Check sheet for the modelled part. Datum: model origin and axes. Units: mm. Face numbers are marked on the shaded views. Coordinates: 2 decimals unless noted, no trailing zeros. Write each loop counter-clockwise with the first axis right and the second up, starting at its lowest first coordinate (ties: lowest second). Pieces come first, ordered by that corner, then holes. Notation, with made-up numbers: (-11.5, -1.5) - (44.5, -1.5) arc R28 ccw to (44.5, 18.5) - close; hole circle Ø10 at (31, -14). An arc over 180 degrees is marked (long way). Write each question's results on one line, items separated by ' | '.
from build123d import *

# Parameters (mm, degrees)
CROQUIS1_R              = 50
CROQUIS1_R_2            = 45
SALIENTE_EXTRUIR1_DEPTH = 400
CROQUIS2_R              = 55
SALIENTE_EXTRUIR2_DEPTH = 30
SALIENTE_EXTRUIR3_START = -30
CROQUIS3_R              = 55
SALIENTE_EXTRUIR3_DEPTH = 30
CROQUIS4_R              = 12.75
CORTAR_EXTRUIR1_DEPTH   = 179
CROQUIS5_R              = 7.5
CROQUIS5_R_2            = 5
CROQUIS5_R_3            = 12.7
CORTAR_EXTRUIR2_DEPTH   = 60


with BuildPart() as part:
    # Croquis1 → Saliente-Extruir1 (new body)
    with BuildSketch(Plane.XY):
        Circle(CROQUIS1_R)
        Circle(CROQUIS1_R_2, mode=Mode.SUBTRACT)
    extrude(amount=SALIENTE_EXTRUIR1_DEPTH)

    # Croquis2 → Saliente-Extruir2 (add)
    with BuildSketch(Plane.XY):
        Circle(CROQUIS2_R)
    extrude(amount=SALIENTE_EXTRUIR2_DEPTH)

    # Croquis3 → Saliente-Extruir3 (add)
    with BuildSketch(Plane.XY.offset(400).offset(SALIENTE_EXTRUIR3_START)):
        Circle(CROQUIS3_R)
    extrude(amount=SALIENTE_EXTRUIR3_DEPTH)

    # Croquis4 → Cortar-Extruir1 (cut)
    with BuildSketch(Plane(origin=(0, 0, 0), x_dir=(0, 0, -1), z_dir=(1, 0, 0))):
        with Locations(Location((-200, 0, 0), (0, 0, 180))):
            Circle(CROQUIS4_R)
    extrude(amount=-CORTAR_EXTRUIR1_DEPTH, mode=Mode.SUBTRACT)

    # Croquis5 → Cortar-Extruir2 (cut)
    with BuildSketch(Plane(origin=(0, 50, 0), x_dir=(1, 0, 0), z_dir=(0, 1, 0))):
        with Locations(Location((0, -240, 0), (0, 0, 270))):
            Circle(CROQUIS5_R)
        with Locations(Location((0, -160, 0), (0, 0, 270))):
            Circle(CROQUIS5_R)
        with Locations(Location((0, -200, 0), (0, 0, 270))):
            Circle(CROQUIS5_R_2)
        with Locations(Location((0, -350, 0), (0, 0, 270))):
            Circle(CROQUIS5_R_3)
        with Locations(Location((0, -50, 0), (0, 0, 270))):
            Circle(CROQUIS5_R_3)
    extrude(amount=-CORTAR_EXTRUIR2_DEPTH, mode=Mode.SUBTRACT)


solid = part.part
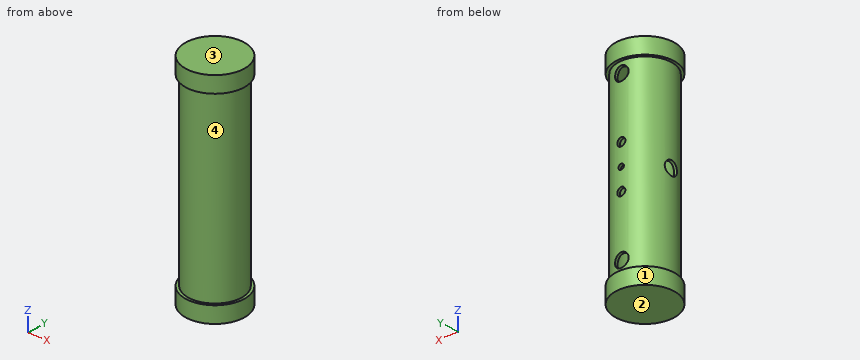
1. Draft check along Z on the marked faces 1, 2, 3 and 4. Enter one of: pulls with the +Z half, pulls with the -Z half, needs draft (parallel to the pull), parting line crosses it, or undercut.
Values follow:
face 1: needs draft | face 2: pulls with the -Z half | face 3: pulls with the +Z half | face 4: undercut
2. Sectioned sample at D-D (z = 98). Record the cut outline in (x, y), then the cut area to 3 significant figures.
Values follow:
outline: circle Ø100 at (0, 0); hole circle Ø90 at (0, 0) | area: 1,490 mm^2
3. Go/stop test with flat-tipped pins: pin 1 (8 mm diameter, centred on x = 0, z = 200, fed in from +Y); pin 2 (12 mm diameter, centred on x = 0, z = 160, fed in from +Y); pin 3 (12 mm diameter, centred on x = -10, y = 29, fed in from -Z); pin 4 (12 mm diameter, centred on y = 42.5, z = 253.5, fed in from +X). Record where each tip stops, or that it passes through.
Values follow:
pin 1: stops at y = -44.82 | pin 2: stops at y = -44.6 | pin 3: stops at z = 0 | pin 4: stops at x = 34.17
4. Sectioned sample at A-A (z = 200). Record the cut outline in (x, y), then the cut area to 3 significant figures.
Values follow:
outline: (-48.35, -12.75) arc R50 ccw (long way) to (5, 49.75) - (5, 44.72) arc R45 cw (long way) to (-43.16, -12.75) - close; (-48.35, 12.75) - (-43.16, 12.75) arc R45 cw to (-5, 44.72) - (-5, 49.75) arc R50 ccw to start | area: 1,310 mm^2
5. Sectioned sample at B-B (y = 21). Record the cut outline in (x, z), then the cut area to 3 significant figures.
Values follow:
outline: (-50.83, 0) - (50.83, 0) - (50.83, 30) - (45.38, 30) - (45.38, 370) - (50.83, 370) - (50.83, 400) - (-50.83, 400) - (-50.83, 370) - (-45.38, 370) - (-45.38, 30) - (-50.83, 30) - close; hole (-39.8, 30) - (39.8, 30) - (39.8, 370) - (-39.8, 370) - close | area: 9,890 mm^2
6. Sectioned sample at C-C (x = 30.5). Record the cut outline in (y, z).
Values follow:
outline: (-45.77, 0) - (45.77, 0) - (45.77, 30) - (39.62, 30) - (39.62, 370) - (45.77, 370) - (45.77, 400) - (-45.77, 400) - (-45.77, 370) - (-39.62, 370) - (-39.62, 30) - (-45.77, 30) - close; hole (-33.09, 30) - (33.09, 30) - (33.09, 370) - (-33.09, 370) - close
7. Material ranges on L1, parallel to Z at x = 5, y = -2; L2, parallel to Z at x = 0, y = 46.9; L3, parallel to X at y = 0, z = 178, recorded low to high. Write a range as [from, to].
Values follow:
L1: z = [0, 30], [370, 400] | L2: z = [0, 37.3], [62.7, 152.5], [167.5, 195], [205, 232.5], [247.5, 337.3], [362.7, 400] | L3: x = [-50, -45], [45, 50]
